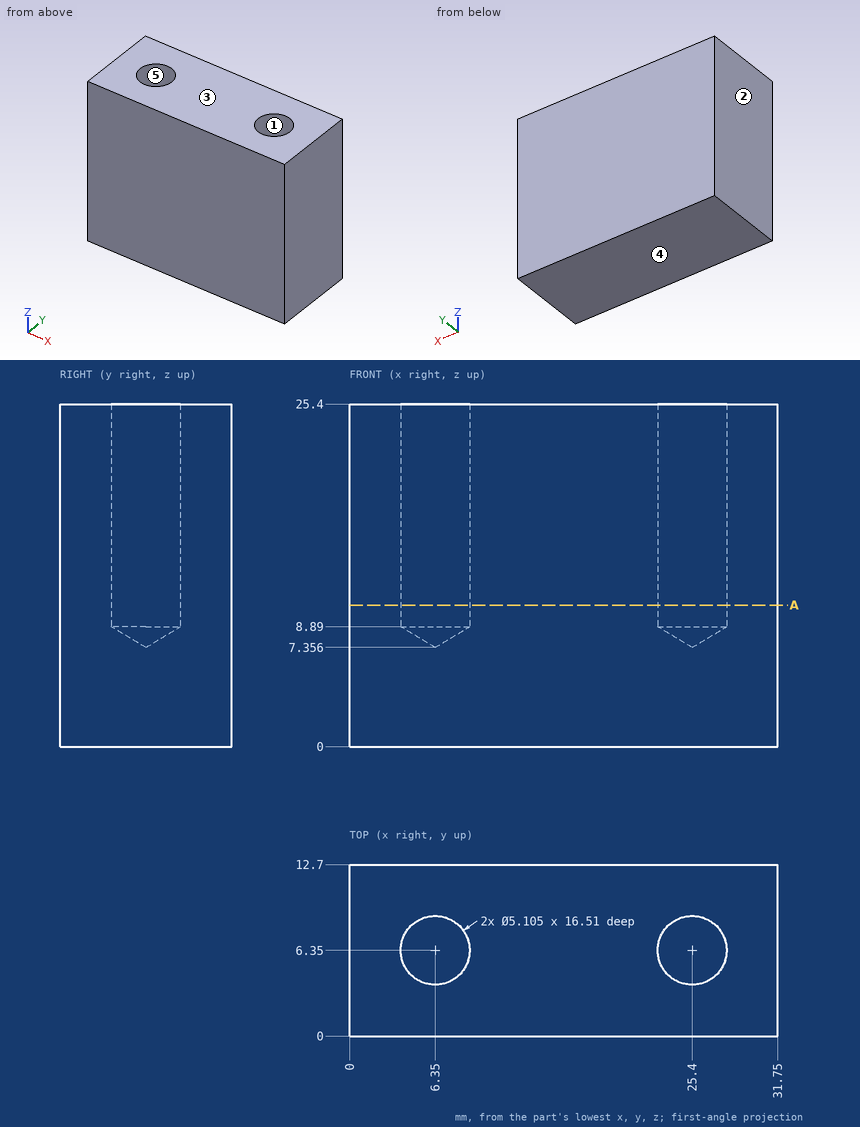
Verification items for this drawing (mm, ordinates from the low corner). A direction names the side the tool comes from. Give positions to 0.01 mm unless a question says otherwise; leave off trailing zeros. Answer as a JSON object with one key per item and string values. Group by question number.
Item 1: Access from +Z, -Z, +X, -X, +Y, -Y to the whole of each face (thin tool, end or side, straight path). Record for the marked faces 1 and 2.
Item 2: Gauge pin test, flat end, axial feed: pin 1 (4.5 mm diameter, centred on x = 6.35, y = 6.35, fed in from +Z). Record the tip position at first contact, or that the pin passes through.
Item 3: Mould release check, pull along Z, two halves, no side actions. Record for the marked faces 3, 4 and 5: pulls with the +Z half, pulls with the -Z half, needs draft (parallel to the pull), parting line crosses it, or undercut.
Item 4: Material ranges on L1, parallel to X at y = 6.35, z = 19.75; L2, parallel to X at y = 8, z = 10.5; L3, parallel to Y at x = 25.4, z = 21.25, recorded low to high.
Item 5: Sectioned sample at A-A on z = 10.5. Give the number of separate pieces and of enclosed holes in the cut face, plus the area to 3 significant figures.
Findings below:
{
 "1": {"face 1": "+Z", "face 2": "+Z, -Z, -X, +Y, -Y"},
 "2": {"pin 1": "z = 8.71"},
 "3": {"face 3": "pulls with the +Z half", "face 4": "pulls with the -Z half", "face 5": "needs draft"},
 "4": {"L1": "0 to 3.8, 8.9 to 22.85, 27.95 to 31.75", "L2": "0 to 4.4, 8.3 to 23.45, 27.35 to 31.75", "L3": "0 to 3.8, 8.9 to 12.7"},
 "5": {"separate pieces": "1", "enclosed holes": "2", "area": "362 mm2"}
}
